```python
from build123d import *

# Parameters (mm, degrees)
ENL_V_MAT_EXTRU_2_DEPTH      = 1
R_P_TITION_CIRCULAIRE1_COUNT = 12
ESQUISSE9_R                  = 16.652952846
ESQUISSE9_R_2                = 16.152952846
ENL_V_MAT_EXTRU_3_DEPTH      = 1
ECHELLE3_SCALE               = 0.6
ESQUISSE12_R                 = 6
BOSS_EXTRU_2_DEPTH           = 10
ESQUISSE13_R                 = 2.75
ENL_V_MAT_EXTRU_5_DEPTH      = 32.69773054


with BuildPart() as part:
    # Esquisse3 → Révolution3 (revolve)
    with BuildSketch(Plane.XY, mode=Mode.PRIVATE) as r_volution3_sk:
        with BuildLine():
            Line((5, 17.5), (5, 16.5))
            ThreePointArc((5, 16.5), (10.181885267, 16.340581134), (15, 14.426653308))
            Line((15, 14.426653308), (20, 14.426653308))
            Line((20, 14.426653308), (20, 12.426653308))
            Line((20, 12.426653308), (18, 12.426653308))
            ThreePointArc((18, 12.426653308), (26.637443378, 8.760216774), (30, 0))
            Line((30, 0), (0, 0))
            Line((0, 0), (0, 17.5))
            Line((0, 17.5), (5, 17.5))
        make_face()
    revolve(r_volution3_sk.sketch.rotate(Axis((-14.762690298, 0, 0), (1, 0, 0)), 90), axis=Axis((-14.762690298, 0, 0), (1, 0, 0)))

    # Esquisse8 → Enlèv. mat.-Extru.2 (cut)
    with BuildSketch(Plane(origin=(0, 0, 0), x_dir=(1, 0, 0), z_dir=(0, 1, 0))):
        with BuildLine():
            Line((5, 16.5), (5, 16))
            ThreePointArc((5, 16), (10.181885267, 15.840581134), (15, 13.926653308))
            Line((15, 13.926653308), (15, 14.426653308))
            ThreePointArc((15, 14.426653308), (10.181885267, 16.340581134), (5, 16.5))
        make_face()
    enl_v_mat_extru_2 = extrude(amount=-ENL_V_MAT_EXTRU_2_DEPTH, mode=Mode.SUBTRACT)

    # Répétition circulaire1: Enlèv. mat.-Extru.2 ×12 about axis
    r_p_tition_circulaire1_axis = Axis((0, 0, 0), (1, 0, 0))
    for i in range(1, R_P_TITION_CIRCULAIRE1_COUNT):
        add(enl_v_mat_extru_2.rotate(r_p_tition_circulaire1_axis, i * 360 / R_P_TITION_CIRCULAIRE1_COUNT), mode=Mode.SUBTRACT)

    # Esquisse9 → Enlèv. mat.-Extru.3 (cut)
    with BuildSketch(Plane(origin=(5, 0, 0), x_dir=(0, 0, -1), z_dir=(1, 0, 0))):
        Circle(ESQUISSE9_R)
        Circle(ESQUISSE9_R_2, mode=Mode.SUBTRACT)
    extrude(amount=ENL_V_MAT_EXTRU_3_DEPTH, mode=Mode.SUBTRACT)


with BuildPart() as part_1:
    # Echelle3: scaled about (0, 0, 0)
    add(part.part.scale(ECHELLE3_SCALE))

    # Esquisse12 → Boss.-Extru.2 (add)
    with BuildSketch(Plane.ZY):
        with Locations(Location((0, 0, 0), (0, 0, 180))):
            Circle(ESQUISSE12_R)
    extrude(amount=BOSS_EXTRU_2_DEPTH)

    # Esquisse13 → Enlèv. mat.-Extru.5 (cut, through all)
    with BuildSketch(Plane.ZY.offset(10)):
        Circle(ESQUISSE13_R)
    extrude(amount=-ENL_V_MAT_EXTRU_5_DEPTH, mode=Mode.SUBTRACT)


solid = part_1.part
```
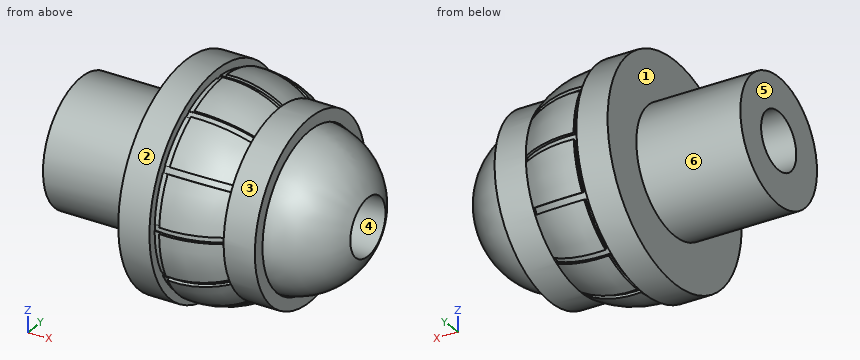
Can you work these out from the model? Positions are in its coordinate system, mm. Face numbers are marked on the shaded views. A direction names the side the tool comes from. Coordinates: 2 decimals unless noted, no trailing zeros. Loops run counter-clockwise (first coordinate to the right, second up) from the corner with the lowest first, then second, coordinate; pieces in that order, holes last.
Item 1: Suppose I cut it at B-B (x = 1.25). Please give me the cut outline in (y, z), then the cut area to 3 significant figures.
Answers below:
outline: circle Ø21 at (0, 0); hole circle Ø5.5 at (0, 0)
area: 323 mm2
Item 2: Which directions (+Z, -Z, +X, -X, +Y, -Y) give clear straight access to the entire face, cutting with the end or side of a thin tool? Please do the marked faces 1, 2 and 3.
Answers below:
face 1: -X
face 2: +X, -X
face 3: +X
Item 3: I'm going to push flat-ended pins straight in: pin 1 (2 mm diameter, centred on x = -1.5, z = 0.5, fed in from +Y); pin 2 (1.5 mm diameter, centred on x = 0, z = -6.5, fed in from +Y); pin 3 (0.6 mm diameter, centred on y = 9.5, z = 2, fed in from -X). Where does each tip first touch, or does it pass through?
Answers below:
pin 1: stops at y = 6
pin 2: stops at y = 8.79
pin 3: stops at x = 0
Item 4: Please list where these lines run through material, in increasing order: L1, parallel to Y at x = 0.5, z = 0; L2, parallel to X at y = 3.75, z = 7; L3, parallel to Y at x = -3.5, z = 0.5.
Answers below:
L1: y = -10.5 to -2.75, 2.75 to 10.5
L2: x = 0 to 12
L3: y = -5.98 to -2.7, 2.7 to 5.98
Item 5: If we mould it in two halves opening along Y, with no side actions, what happens to the marked faces 4, 5 and 6? For each: released by +Y, released by -Y, zero draft, split by the parting line, or undercut.
Answers below:
face 4: undercut
face 5: zero draft
face 6: split by the parting line
Item 6: Suppose I cut it at A-A (x = -6). Please give me the cut outline in (y, z), then the cut area to 3 significant figures.
Answers below:
outline: circle Ø12 at (0, 0); hole circle Ø5.5 at (0, 0)
area: 89.3 mm2
